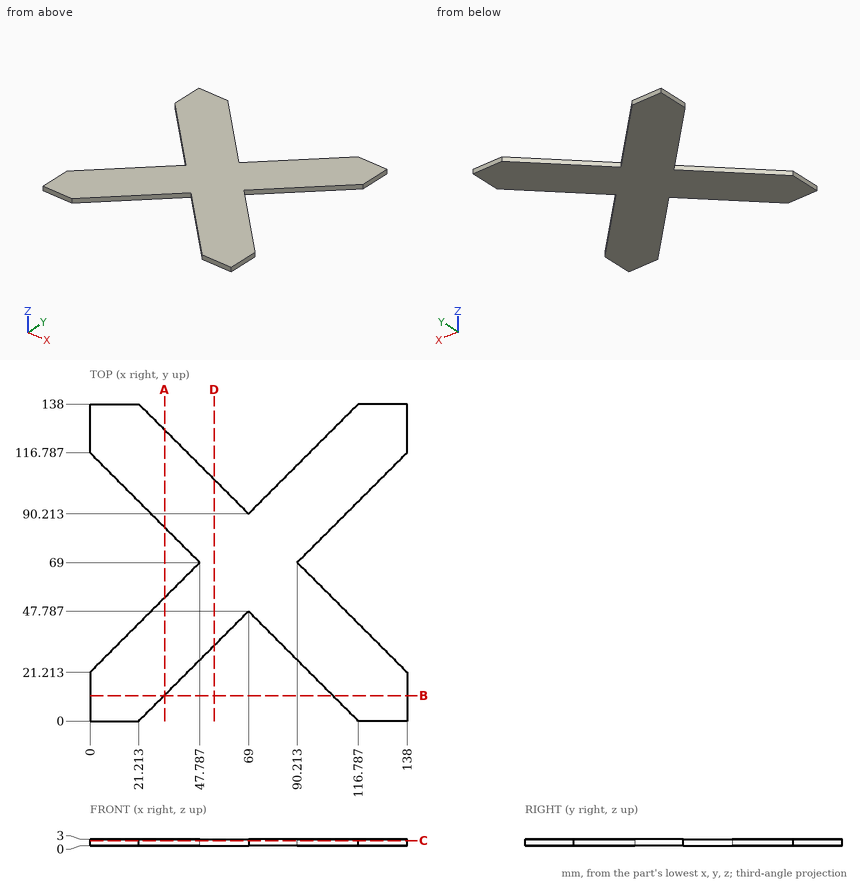
Check sheet for the drawn part. Datum: minimum x, y, z corner. Units: mm. Give positions to 0.01 mm unless a question says otherwise; leave off trailing zeros. Write each loop counter-clockwise with the first axis right and the second up, starting at its lowest first coordinate (ties: lowest second). Pieces come first, ordered by that corner, then holes.
(1) Cross-section at A-A (x = 32.5). Enter the section's corners in (y, z).
(2) Cross-section at B-B (y = 11). Enter the section's corners in (x, z), plus the area to 3 significant figures.
(3) Cross-section at D-D (x = 54). Enter the section's corners in (y, z).
(4) Material ranges on line 1 (Y direction, x = 101.5, z = 0.4); line 2 (X direction, y = 118, z = 2.55); line 3 (Y direction, x = 91, z = 1), recorded low to high.
(5) Gauge pin test, flat end, axial feed: pin 1 (1.5 mm diameter, centred on y = 44, z = 0.5, fed in from +X). Record the tip position at first contact, or that the pin passes through.
(6) Cross-section at C-C (z = 2.3). Enter the section's corners in (x, y).
Worked out:
1. outline: (11.29, 0) - (53.71, 0) - (53.71, 3) - (11.29, 3) - close; (84.29, 0) - (126.71, 0) - (126.71, 3) - (84.29, 3) - close
2. outline: (0, 0) - (32.21, 0) - (32.21, 3) - (0, 3) - close; (105.79, 0) - (138, 0) - (138, 3) - (105.79, 3) - close
2. area: 193 mm2
3. outline: (32.79, 0) - (105.21, 0) - (105.21, 3) - (32.79, 3) - close
4. line 1: y = 15.29 to 57.71, 80.29 to 122.71
4. line 2: x = 0 to 41.21, 96.79 to 138
4. line 3: y = 25.79 to 68.21, 69.79 to 112.21
5. pin 1: stops at x = 115.96
6. outline: (0, 0) - (21.21, 0) - (69, 47.79) - (116.79, 0) - (138, 0) - (138, 21.21) - (90.21, 69) - (138, 116.79) - (138, 138) - (116.79, 138) - (69, 90.21) - (21.21, 138) - (0, 138) - (0, 116.79) - (47.79, 69) - (0, 21.21) - close
